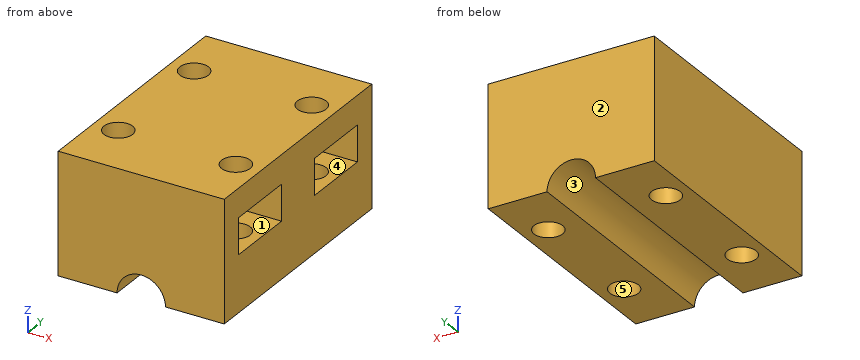
```python
from build123d import *

# Parameters (mm, degrees)
SKETCH1_W               = 48
SKETCH1_H               = 35
BOSS_EXTRUDE1_DEPTH     = 70
SKETCH2_W               = 10.4
SKETCH2_H               = 20.4
CUT_EXTRUDE1_DEPTH      = 45
SKETCH3_R               = 4.15
CUT_EXTRUDE2_DEPTH      = 36
CUT_EXTRUDE3_DEPTH      = 1
CUT_EXTRUDE3_DEPTH_BACK = 71


with BuildPart() as part:
    # Sketch1 → Boss-Extrude1 (new body)
    with BuildSketch(Plane(origin=(0, 0, 0), x_dir=(1, 0, 0), z_dir=(0, 1, 0))):
        Rectangle(SKETCH1_W, SKETCH1_H)
    extrude(amount=BOSS_EXTRUDE1_DEPTH)

    # Sketch2 → Cut-Extrude1 (cut)
    with BuildSketch(Plane(origin=(24, 0, 0), x_dir=(0, 0, -1), z_dir=(1, 0, 0))):
        with Locations((-4, 53)):
            Rectangle(SKETCH2_W, SKETCH2_H)
        with Locations((-4, 17)):
            Rectangle(SKETCH2_W, SKETCH2_H)
    extrude(amount=-CUT_EXTRUDE1_DEPTH, mode=Mode.SUBTRACT)

    # Sketch3 → Cut-Extrude2 (cut, through all)
    with BuildSketch(Plane.XY.offset(17.5)):
        with Locations((17, 53)):
            Circle(SKETCH3_R)
        with Locations((-17, 53)):
            Circle(SKETCH3_R)
        with Locations((-17, 17)):
            Circle(SKETCH3_R)
        with Locations((17, 17)):
            Circle(SKETCH3_R)
    extrude(amount=-CUT_EXTRUDE2_DEPTH, mode=Mode.SUBTRACT)

    # Sketch4 → Cut-Extrude3 (cut, two sides)
    with BuildSketch(Plane(origin=(0, 70, 0), x_dir=(1, 0, 0), z_dir=(0, 1, 0))) as cut_extrude3_sk:
        with BuildLine():
            Line((-7, 121.00935782), (-7, 17.5))
            ThreePointArc((-7, 17.5), (0, 10.5), (7, 17.5))
            Line((7, 17.5), (7, 121.00935782))
            Line((7, 121.00935782), (7, 328.028073461))
            Line((7, 328.028073461), (-7, 328.028073461))
            Line((-7, 328.028073461), (-7, 121.00935782))
        make_face()
    extrude(amount=CUT_EXTRUDE3_DEPTH, mode=Mode.SUBTRACT)
    extrude(cut_extrude3_sk.sketch, amount=-CUT_EXTRUDE3_DEPTH_BACK, mode=Mode.SUBTRACT)


solid = part.part
```
Check sheet for the modelled part. Datum: model origin and axes. Units: mm. Face numbers are marked on the shaded views. A direction names the side the tool comes from. Round coordinates to 2 decimals unless told otherwise and drop trailing zeros. Order: outer loops, then holes, each group sorted by start corner. A loop starts at its lowest first (then second) coordinate and runs counter-clockwise, first axis right, second up.
1) Tool access check on the marked faces 4 and 5. Record the directions out of +Z, -Z, +X, -X, +Y, -Y that give a thin tool (end or side, any length) a straight path to the whole face; none if there is none.
2) Section check D-D (x = 0). Record the boundary of the cut face in (y, z), and give its area (3 significant figures).
3) Section check A-A (x = -17). Record the boundary of the cut face in (y, z), and give its area (3 significant figures).
4) Scan lines: line 1 (Y direction, x = -19, z = 8); line 2 (Y direction, x = 17, z = 13); line 3 (Z direction, x = 8, y = 43.5). Record each from-to range of solid material in increasing order.
5) Section check C-C (z = 14). Record the boundary of the cut face in (x, y).
6) Section check B-B (y = 53). Record the boundary of the cut face in (x, z), and give its area (3 significant figures).
7) Mould release check, pull along Y, two halves, no side actions. Record for the marked faces 1, 2 and 3: +Y half, -Y half, draft (parallel to the pull), parting line (faces both ways), or undercut.
8) Go/stop test with flat-tipped pins: pin 1 Ø4.5 at (y, z) = (24.5, 5.5) entering from +X; pin 2 Ø6 at (x, y) = (1, 15.5) entering from -Z. Record where each tip stops, or that it passes through.
Result:
1. face 4: +X
1. face 5: +Z, -Z
2. outline: (0, -10.5) - (70, -10.5) - (70, 17.5) - (0, 17.5) - close; hole (6.8, -1.2) - (27.2, -1.2) - (27.2, 9.2) - (6.8, 9.2) - close; hole (42.8, -1.2) - (63.2, -1.2) - (63.2, 9.2) - (42.8, 9.2) - close
2. area: 1,540 mm2
3. outline: (0, -17.5) - (12.85, -17.5) - (12.85, -1.2) - (6.8, -1.2) - (6.8, 9.2) - (12.85, 9.2) - (12.85, 17.5) - (0, 17.5) - close; (21.15, -17.5) - (48.85, -17.5) - (48.85, -1.2) - (42.8, -1.2) - (42.8, 9.2) - (48.85, 9.2) - (48.85, 17.5) - (21.15, 17.5) - (21.15, 9.2) - (27.2, 9.2) - (27.2, -1.2) - (21.15, -1.2) - close; (57.15, -17.5) - (70, -17.5) - (70, 17.5) - (57.15, 17.5) - (57.15, 9.2) - (63.2, 9.2) - (63.2, -1.2) - (57.15, -1.2) - close
3. area: 1,620 mm2
4. line 1: y = 0 to 6.8, 27.2 to 42.8, 63.2 to 70
4. line 2: y = 0 to 12.85, 21.15 to 48.85, 57.15 to 70
4. line 3: z = -17.5 to -1.2, 9.2 to 17.5
5. outline: (-24, 0) - (24, 0) - (24, 70) - (-24, 70) - close; hole circle Ø8.3 at (-17, 17); hole circle Ø8.3 at (-17, 53); hole circle Ø8.3 at (17, 17); hole circle Ø8.3 at (17, 53)
6. outline: (-24, -17.5) - (-21.15, -17.5) - (-21.15, 17.5) - (-24, 17.5) - close; (-12.85, -17.5) - (-7, -17.5) arc R7 cw to (7, -17.5) - (12.85, -17.5) - (12.85, -1.2) - (-12.85, -1.2) - close; (-12.85, 9.2) - (12.85, 9.2) - (12.85, 17.5) - (-12.85, 17.5) - close; (21.15, -17.5) - (24, -17.5) - (24, -1.2) - (21.15, -1.2) - close; (21.15, 9.2) - (24, 9.2) - (24, 17.5) - (21.15, 17.5) - close
6. area: 725 mm2
7. face 1: undercut
7. face 2: +Y half
7. face 3: draft
8. pin 1: stops at x = -21
8. pin 2: stops at z = -11.76
